The model under review builds one solid part; all positions refer to its coordinate system, in mm. A direction names the side the tool comes from. Coordinates: 2 decimals unless noted, no trailing zeros. Write each loop counter-clockwise with the first axis right and the second up, starting at its lowest first coordinate (ties: lowest second). Pieces come first, ordered by that corner, then holes.
```python
from build123d import *

# Parameters (mm, degrees)
F1_DEPTH = 16.891
F3_DEPTH = 6.35
F5_DEPTH = 6.35


with BuildPart() as f1:
    # F0 (on Front) → F1 (new body)
    with BuildSketch(Plane.XZ):
        Polygon((0, 6.35), (0, 0), (6.35, 0), (26.416, 0), (26.416, 6.35), (6.35, 6.35), (6.35, 26.416), (0, 26.416), align=None)
    extrude(amount=F1_DEPTH)

    # F2 (on face) → F3 (cut, through all)
    with BuildSketch(Plane.YZ.offset(6.35)):
        with BuildLine():
            Line((-8.4455, 16.383), (-3.7465, 16.383))
            ThreePointArc((-3.7465, 16.383), (-5.122805, 19.705695), (-8.4455, 21.082))
            Line((-8.4455, 21.082), (-8.4455, 16.383))
        make_face()
        with BuildLine():
            ThreePointArc((-8.4455, 11.684), (-5.122805, 13.060305), (-3.7465, 16.383))
            Line((-3.7465, 16.383), (-8.4455, 16.383))
            Line((-8.4455, 16.383), (-8.4455, 11.684))
        make_face()
        with BuildLine():
            Line((-8.4455, 16.383), (-8.4455, 21.082))
            ThreePointArc((-8.4455, 21.082), (-11.768195, 19.705695), (-13.1445, 16.383))
            Line((-13.1445, 16.383), (-8.4455, 16.383))
        make_face()
        with BuildLine():
            ThreePointArc((-13.1445, 16.383), (-11.768195, 13.060305), (-8.4455, 11.684))
            Line((-8.4455, 11.684), (-8.4455, 16.383))
            Line((-8.4455, 16.383), (-13.1445, 16.383))
        make_face()
    extrude(amount=-F3_DEPTH, mode=Mode.SUBTRACT)

    # F4 (on face) → F5 (cut, through all)
    with BuildSketch(Plane.XY.offset(6.35)):
        with BuildLine():
            Line((16.383, -8.4455), (21.082, -8.4455))
            ThreePointArc((21.082, -8.4455), (19.705695, -5.122805), (16.383, -3.7465))
            Line((16.383, -3.7465), (16.383, -8.4455))
        make_face()
        with BuildLine():
            ThreePointArc((16.383, -13.1445), (19.705695, -11.768195), (21.082, -8.4455))
            Line((21.082, -8.4455), (16.383, -8.4455))
            Line((16.383, -8.4455), (16.383, -13.1445))
        make_face()
        with BuildLine():
            Line((16.383, -8.4455), (16.383, -3.7465))
            ThreePointArc((16.383, -3.7465), (13.060305, -5.122805), (11.684, -8.4455))
            Line((11.684, -8.4455), (16.383, -8.4455))
        make_face()
        with BuildLine():
            ThreePointArc((11.684, -8.4455), (13.060305, -11.768195), (16.383, -13.1445))
            Line((16.383, -13.1445), (16.383, -8.4455))
            Line((16.383, -8.4455), (11.684, -8.4455))
        make_face()
    extrude(amount=-F5_DEPTH, mode=Mode.SUBTRACT)


solid = f1.part
```
Item 1: Take a section at A-A, the plane x = 5.5. Write out the cut boundary in (y, z), plus the area to 3 significant figures.
Solved:
outline: (-16.89, 0) - (0, 0) - (0, 26.42) - (-16.89, 26.42) - close; hole (-13.14, 16.38) arc R4.7 ccw to (-8.45, 11.68) arc R4.7 ccw to (-3.75, 16.38) arc R4.7 ccw to (-8.45, 21.08) arc R4.7 ccw to start
area: 377 mm2
Item 2: Machinability: for faces 1 (the face through (4, -16.891, 8)), 2 (the face through (6.35, -6, 12)), which of the approach directions +Z, -Z, +X, -X, +Y, -Y give a long, thin tool a straight path to every point of the face, cutting with its end or side? Answer none if there is none.
Solved:
face 1: +Z, -Z, +X, -X, -Y
face 2: +Z, +X, +Y, -Y
Item 3: Take a section at B-B, the plane z = 3.5. Write out the cut boundary in (x, y), plus the area to 3 significant figures.
Solved:
outline: (0, -16.89) - (26.42, -16.89) - (26.42, 0) - (0, 0) - close; hole (11.68, -8.45) arc R4.7 ccw to (16.38, -13.14) arc R4.7 ccw to (21.08, -8.45) arc R4.7 ccw to (16.38, -3.75) arc R4.7 ccw to start
area: 377 mm2
Item 4: Take a section at D-D, the plane x = 14. Write out the cut boundary in (y, z).
Solved:
outline: (-16.89, 0) - (-12.5, 0) - (-12.5, 6.35) - (-16.89, 6.35) - close; (-4.4, 0) - (0, 0) - (0, 6.35) - (-4.4, 6.35) - close
Item 5: For pin 1 (8.5 mm diameter, centred on x = 15, y = -10, fed in from +Z); pin 2 (5 mm diameter, centred on y = -14.5, z = 23.5, fed in from +X), all flat-tipped, find the tip position at first contact; note any pin that passes through.
Solved:
pin 1: stops at z = 6.35
pin 2: stops at x = 6.35
Item 6: Take a section at C-C, the plane y = -7.5. Write out the cut boundary in (x, z).
Solved:
outline: (0, 0) - (11.78, 0) - (11.78, 6.35) - (6.35, 6.35) - (6.35, 11.78) - (0, 11.78) - close; (0, 20.99) - (6.35, 20.99) - (6.35, 26.42) - (0, 26.42) - close; (20.99, 0) - (26.42, 0) - (26.42, 6.35) - (20.99, 6.35) - close
Item 7: To check wall thickness, follow line 1 along X through (y, z) = (-3.25, 9.5); line 2 along Y through (x, z) = (5.75, 20.5). State the ranges of each line that lie inside material, in increasing order.
Solved:
line 1: x = 0 to 6.35
line 2: y = -16.89 to -10.71, -6.18 to 0
